Could you check a few things on this model? Use its own coordinates, in mm. Round coordinates to 2 decimals unless told otherwise and drop trailing zeros. Loops run counter-clockwise (first coordinate to the right, second up) from the corner with the lowest first, then second, coordinate; pieces in that order, holes last. Notation, with made-up numbers: (17, 62.25) -> (30, 62.25) arc R7 ccw to (30, 66.25) -> close; hole circle Ø2 at (69, 21.5). An arc over 180 degrees is marked (long way). One line per item, written item: value.
```python
from build123d import *

# Parameters (mm, degrees)
F0_R     = 47.625
F1_DEPTH = 3.429


# Not quite as in the source:
# - ends of sketch curves that miss each other by under 0.0002 mm in the source are joined


with BuildPart() as f1:
    # F0 (on Front) → F1 (new body)
    with BuildSketch(Plane.XZ):
        with BuildLine():
            Line((-235.938695, 504.0320628), (-209.655918, 446.5764754))
            Line((-209.655918, 446.5764754), (-152.505918, 446.5764754))
            Line((-152.505918, 446.5764754), (-126.223141, 504.0320628))
            ThreePointArc((-126.223141, 504.0320628), (-181.080918, 589.4514754), (-235.938695, 504.0320628))
        make_face()
        with Locations((-181.080918, 529.1264754)):
            Circle(F0_R, mode=Mode.SUBTRACT)
    extrude(amount=F1_DEPTH)


solid = f1.part
```
Item 1: If we section it at A-A on x = -157.5: List the corners of the cut face in (y, z) for me, plus the area to 3 significant figures.
Output:
outline: (-3.43, 446.58) -> (0, 446.58) -> (0, 487.75) -> (-3.43, 487.75) -> close; (-3.43, 570.5) -> (0, 570.5) -> (0, 584.65) -> (-3.43, 584.65) -> close
area: 190 mm²
Item 2: I need wall thicknesses on line 1 (Z direction, x = -182.5, y = -1.6); line 2 (X direction, y = -2.5, z = 529); line 3 (X direction, y = -2.45, z = 495). Which ranges of each line are inside material? Lowest first, please. Write a range as from..to.
Output:
line 1: z = 446.58..481.52, 576.73..589.43
line 2: x = -241.41..-228.71, -133.46..-120.76
line 3: x = -231.81..-214.3, -147.86..-130.35
Item 3: If we section it at C-C on y = -2.5: List the corners of the cut face in (x, z) for me (3 decimals).
Output:
outline: (-235.939, 504.032) -> (-209.656, 446.576) -> (-152.506, 446.576) -> (-126.223, 504.032) arc R60.325 ccw (long way) to start; hole circle Ø95.25 at (-181.081, 529.126)
Item 4: If we mould it in two halves opening along X, with no side actions, what happens to faces 1 (the face through (-222.981, -1.69, 475.706)), 2 (the face through (-155, 0, 487)), 3 (the face through (-187.281, -1.69, 576.346))? For each: released by +X, released by -X, zero draft, split by the parting line, or undercut.
Output:
face 1: released by -X
face 2: zero draft
face 3: undercut
Item 5: If we section it at D-D on z = 473: List the corners of the cut face in (x, y) for me.
Output:
outline: (-221.74, -3.43) -> (-140.42, -3.43) -> (-140.42, 0) -> (-221.74, 0) -> close
Item 6: Will these pins go through, and if not, where does the flat tip stop? pin 1 Ø2 at (y, z) = (-1.5, 518.5) entering from -X; pin 2 Ø2 at (y, z) = (-1, 524.5) entering from +X (3 decimals); pin 3 Ø1.5 at (y, z) = (-1.5, 561) entering from +X.
Output:
pin 1: stops at x = -240.63
pin 2: stops at x = -120.865
pin 3: stops at x = -129.4
Item 7: If we section it at B-B on z = 490: List the corners of the cut face in (x, y) for me.
Output:
outline: (-229.52, -3.43) -> (-208.23, -3.43) -> (-208.23, 0) -> (-229.52, 0) -> close; (-153.93, -3.43) -> (-132.64, -3.43) -> (-132.64, 0) -> (-153.93, 0) -> close
